Autodesk Inventor part; units mm, degrees
ref_plane "YZ Plane" through (0, 0, 0) normal (1, 0, 0) x (0, 1, 0)
ref_plane "XZ Plane" through (0, 0, 0) normal (0, 1, 0) x (-1, 0, 0)
ref_plane "XY Plane" through (0, 0, 0) normal (0, 0, 1) x (1, 0, 0)
sketch "Sketch1" plane through (0, 0, 0) normal (1, 0, 0) x (0, 1, 0)
  line L0 (0, 0) -> (98.425, 0)
  line L1 (98.425, 0) -> (98.425, -107.95)
  line L2 (98.425, -107.95) -> (0, -107.95)
  line L3 (0, -107.95) -> (0, 0)
  line L4 (0, -1.905) -> (-3.175, -1.905)
  line L5 (-3.175, -1.905) -> (-3.175, -32.385)
  line L6 (-3.175, -32.385) -> (0, -32.385)
  line L7 (0, -32.385) -> (0, -1.905)
  line L8 (0, -75.565) -> (-3.175, -75.565)
  line L9 (-3.175, -75.565) -> (-3.175, -106.045)
  line L10 (-3.175, -106.045) -> (0, -106.045)
  line L11 (0, -106.045) -> (0, -75.565)
  dimension "d0" = 107.95
  dimension "d1" = 3.175
  dimension "d2" = 3.175
  dimension "d3" = 30.48
  dimension "d4" = 30.48
  dimension "d5" = 1.905
  dimension "d6" = 1.905
  dimension "d7" = 98.425
extrude "Extrusion1" add sketch "Sketch1" along normal blind 3.175
sketch "Sketch2" plane through (3.175, 0, 0) normal (1, 0, 0) x (0, 0, -1)
  line L0 (101.6, 49.149) -> (81.28, 49.149)
  line L1 (81.28, 49.149) -> (81.28, 8.89)
  line L2 (81.28, 8.89) -> (101.6, 8.89)
  line L3 (101.6, 8.89) -> (101.6, 49.149)
  line L4 (32.385, 0) -> (75.565, 0)
  line L5 (0, 98.425) -> (0, 0)
  line L6 (107.95, 0) -> (107.95, 98.425)
  dimension "d10" = 40.259
  dimension "d11" = 20.32
  dimension "d12" = 8.89
  dimension "d14" = 6.35
extrude "Extrusion2" cut sketch "Sketch2" against normal blind 3.175
sketch "Sketch3" plane through (3.175, 0, 0) normal (1, 0, 0) x (0, 0, -1)
  point P0 (0, 0)
sketch "Sketch4" plane through (3.175, 0, 0) normal (1, 0, 0) x (0, 0, -1)
  line L0 (-26.3959, 105.0556) -> (55.1146, 105.0556)
  line L1 (55.1146, 105.0556) -> (55.1146, 12.1421)
  line L2 (55.1146, 12.1421) -> (-26.3959, 12.1421)
  line L3 (-26.3959, 12.1421) -> (-26.3959, 105.0556)
  point P0 (0, 0)
extrude "Extrusion3" cut sketch "Sketch4" against normal blind 3.175
sketch "Sketch5" plane through (3.175, 0, 0) normal (1, 0, 0) x (0, 0, -1)
  circle A0 centre (73.7235, 70.2891) radius 1.651
  circle A1 centre (89.3445, 70.2891) radius 1.651
  line L0 (107.95, 0) -> (107.95, 98.425)
  point P0 (0, 0)
  dimension "d19" = 3.302
  dimension "d20" = 3.302
  dimension "d21" = 15.621
  dimension "d22" = 18.6055
  dimension "d23" = 0
extrude "Extrusion4" cut sketch "Sketch5" against normal blind 3.175
properties part number "rib"
Verification items for the finished model (mm, model axes). A direction names the side the tool comes from. Coordinates: 2 decimals unless noted, no trailing zeros. Loops run counter-clockwise (first coordinate to the right, second up) from the corner with the lowest first, then second, coordinate; pieces in that order, holes last. Notation, with made-up numbers: (-24, -19.5) -> (30, -19.5) arc R22 ccw to (30, 9.5) -> close; hole circle Ø1 at (-15.75, 18.25). An arc over 180 degrees is marked (long way). Answer as a JSON object with one key per item and string values. Group by question number.
Item 1: Sectioned sample at A-A on z = -93.5. Record the boundary of the cut face in (x, y) (3 decimals), plus the area to 3 significant figures.
Item 2: Sectioned sample at D-D on y = 80. Record the boundary of the cut face in (x, z) (3 decimals).
Item 3: Depth check by flat-ended pin: pin 1 (1.6 mm diameter, centred on x = 1.5, y = -2, fed in from -Z) (3 decimals); pin 2 (2 mm diameter, centred on y = 17.5, z = -55.5, fed in from -X); pin 3 (0.6 mm diameter, centred on x = 2.5, z = -107, fed in from -Y); pin 4 (1.6 mm diameter, centred on x = 2, y = 28.5, fed in from +Z). Enter the tip coordinate at first touch or a pass-through.
Item 4: Mould release check, pull along Z, two halves, no side actions. Record for faces 1 (the flat face through (2, 29, -81.28)), 2 (the flat face through (2, 50, -107.95)), 3 (the flat face through (2, 12.142, -28)): +Z half, -Z half, draft (parallel to the pull), parting line (faces both ways), or undercut.
Item 5: Sectioned sample at C-C on x = 1.4. State how many separate pieces and enclosed holes the cut face has, plus the area to 3 significant figures.
Item 6: Scan lines: probe 1 along Y at (x, z) = (1.95, -81.5) (3 decimals); probe 2 along Z at (x, y) = (2.8, 70); probe 3 along Z at (x, y) = (1.5, 19.5). Record each from-to range of solid material in increasing order.
Item 7: Tool access check on faces 4 (the flat face through (2, 6, 0)), 5 (the flat face through (2, -2, -32.385)), 6 (the flat face through (2, 56, -55.115)), 7 (the flat face through (2, -2, -1.905)), 8 (the flat face through (2, 8.89, -91)). Record the directions out of +Z, -Z, +X, -X, +Y, -Y that give a thin tool (end or side, any length) a straight path to the whole face; none if there is none.
Item 8: Sectioned sample at B-B on y = 32.5. Record the boundary of the cut face in (x, z) (3 decimals).
Evaluation:
{
 "1": {"outline": "(0, -3.175) -> (3.175, -3.175) -> (3.175, 8.89) -> (0, 8.89) -> close; (0, 49.149) -> (3.175, 49.149) -> (3.175, 98.425) -> (0, 98.425) -> close", "area": "195 mm²"},
 "2": {"outline": "(0, -107.95) -> (3.175, -107.95) -> (3.175, -55.115) -> (0, -55.115) -> close"},
 "3": {"pin 1": "stops at z = -106.045", "pin 2": "stops at x = 0", "pin 3": "stops at y = 0", "pin 4": "stops at z = -55.11"},
 "4": {"face 1": "undercut", "face 2": "-Z half", "face 3": "draft"},
 "5": {"separate pieces": "1", "enclosed holes": "3", "area": "5,230 mm²"},
 "6": {"probe 1": "y = -3.175 to 8.89, 49.149 to 98.425", "probe 2": "z = -107.95 to -90.97, -87.72 to -75.35, -72.1 to -55.11", "probe 3": "z = -107.95 to -101.6, -81.28 to -55.11"},
 "7": {"face 4": "+Z, +X, -X, +Y, -Y", "face 5": "+X, -X, -Y", "face 6": "+Z, +X, -X, +Y", "face 7": "+Z, +X, -X, -Y", "face 8": "+X, -X"},
 "8": {"outline": "(0, -107.95) -> (3.175, -107.95) -> (3.175, -101.6) -> (0, -101.6) -> close; (0, -81.28) -> (3.175, -81.28) -> (3.175, -55.115) -> (0, -55.115) -> close"}
}
